```python
from build123d import *

# Parameters (mm, degrees)
F0_R          = 40
F1_DEPTH      = 20
F2_W          = 11
F2_H          = 10
F3_DEPTH      = 50
F3_DEPTH_BACK = 10
F4_R          = 6
F6_DEPTH      = 5
F7_R          = 6.4
F8_DEPTH      = 25
F9_R          = 1.5
F10_DEPTH     = 16
F11_R         = 3
F12_DEPTH     = 6


# Not quite as in the source:
# - a pattern or mirror of a feature is missing from the dataset's text; its kind, count and spacing are read off the source's solid


with BuildPart() as f1:
    # F0 (on Front) → F1 (new body)
    with BuildSketch(Plane.XZ):
        Circle(F0_R)
    extrude(amount=F1_DEPTH)

    # F2 (on Right) → F3 (cut, two sides)
    with BuildSketch(Plane.YZ) as f3_sk:
        with Locations((-5.5, 29)):
            Rectangle(F2_W, F2_H)
    f3 = extrude(amount=F3_DEPTH, mode=Mode.SUBTRACT) + extrude(f3_sk.sketch, amount=-F3_DEPTH_BACK, mode=Mode.SUBTRACT)

    # F3_copies: F3 across plane
    add(f3.mirror(Plane(origin=(0, 0, 0), x_dir=(-1, 0, 0), z_dir=(0, 0, -1))), mode=Mode.SUBTRACT)

    # F4
    f4_edges = [f1.edges().sort_by_distance(p)[0] for p in [
        (-40, -20, 0),
    ]]
    fillet(f4_edges, radius=F4_R)

    # F5 (on face) → F6 (cut)
    with BuildSketch(Plane.XZ.offset(20)):
        Polygon((-5.715767665, -9.9), (5.715767665, -9.9), (11.43153533, 0), (5.715767665, 9.9), (-5.715767665, 9.9), (-11.43153533, 0), align=None)
    extrude(amount=-F6_DEPTH, mode=Mode.SUBTRACT)

    # F7 (on face) → F8 (cut)
    with BuildSketch(Plane.XZ.offset(15)):
        Circle(F7_R)
    extrude(amount=-F8_DEPTH, mode=Mode.SUBTRACT)

    # F9 (on Front) → F10 (cut)
    with BuildSketch(Plane.XZ):
        with Locations((26, 12)):
            Circle(F9_R)
        with Locations((-26, 12)):
            Circle(F9_R)
        with Locations((-26, -12)):
            Circle(F9_R)
        with Locations((26, -12)):
            Circle(F9_R)
    extrude(amount=F10_DEPTH, mode=Mode.SUBTRACT)

    # F11 (on face) → F12 (cut)
    with BuildSketch(Plane(origin=(0, 0, 0), x_dir=(-1, 0, 0), z_dir=(0, 1, 0))):
        with Locations((-26, 12)):
            Circle(F11_R)
        with Locations((26, 12)):
            Circle(F11_R)
        with Locations((26, -12)):
            Circle(F11_R)
        with Locations((-26, -12)):
            Circle(F11_R)
    extrude(amount=-F12_DEPTH, mode=Mode.SUBTRACT)


solid = f1.part
```
The listing builds one solid part. Answer for the finished solid, in the listing's coordinates (mm). A direction names the side the tool comes from. Coordinates: 2 decimals unless noted, no trailing zeros. Loops run counter-clockwise (first coordinate to the right, second up) from the corner with the lowest first, then second, coordinate; pieces in that order, holes last. Notation, with made-up numbers: (3.25, -25.5) -> (21.25, -25.5) arc R34 cw to (21.25, 8.5) -> close; hole circle Ø6 at (87.25, 9). An arc over 180 degrees is marked (long way). Return JSON: item names as keys, results as strings. Group by question number.
(1) Which of the six approach directions +Z, -Z, +X, -X, +Y, -Y give full straight-line access (tool end or side, diameter ignored) to faces 1 (the cylindrical face through (-5.08, -7.6, -3.89)), 2 (the flat face through (11, -6, -24)), 3 (the flat face through (-1, 0, -8)), 4 (the flat face through (8.534, -17.535, -5.019)), 5 (the cylindrical face through (-27.5, -10.93, -11.93))?
(2) Given pin 1 Ø2.5 at (x, z) = (-26, 12) entering from +Y; pin 2 Ø3.5 at (x, z) = (26, 12) entering from +Y; pin 3 Ø3 at (x, z) = (14.5, -26.5) entering from +Y, each flat-ended and moving along its own axis, determine where each tip first touches the part or whether it passes through.
(3) Determine the mould class of faces 6 (the flat face through (24.7, -6, -13.3)), 7 (the flat face through (-10, -6, -29)), 8 (the flat face through (7, -20, 8)) for opening direction X: released by +X, released by -X, zero draft, split by the parting line, or undercut.
(4) A cutting plane is placed at A-A on x = 0. Write down the section's boundary in (y, z).
(5) Find the intervals of material crossed by probe 1 along Z at (x, y) = (26, -3.05); probe 2 along Z at (x, y) = (-4, -4); probe 3 along X at (y, z) = (-14, 12), in increasing order. Write a range as from..to.
(6) A cutting plane is placed at B-B on y = -9.5. Write down the section's boundary in (x, z).
The answers:
{
 "1": {"face 1": "+Y, -Y", "face 2": "+X, +Y", "face 3": "+Z, -Z, +X, -X, +Y", "face 4": "-Y", "face 5": "+Y"},
 "2": {"pin 1": "stops at y = -16", "pin 2": "stops at y = -6", "pin 3": "stops at y = -11"},
 "3": {"face 6": "undercut", "face 7": "released by +X", "face 8": "zero draft"},
 "4": {"outline": "(-20, -34) arc R6 ccw to (-14, -40) -> (0, -40) -> (0, -34) -> (-11, -34) -> (-11, -24) -> (0, -24) -> (0, -6.4) -> (-15, -6.4) -> (-15, -9.9) -> (-20, -9.9) -> close; (-20, 9.9) -> (-15, 9.9) -> (-15, 6.4) -> (0, 6.4) -> (0, 24) -> (-11, 24) -> (-11, 34) -> (0, 34) -> (0, 40) -> (-14, 40) arc R6 ccw to (-20, 34) -> close"},
 "5": {"probe 1": "z = -24..-15, -9..9, 15..24", "probe 2": "z = -39.8..-34, -24..-5, 5..24, 34..39.8", "probe 3": "x = -38.16..-27.5, -24.5..24.5, 27.5..38.16"},
 "6": {"outline": "(-10, -34) -> (-10, -24) -> (32, -24) arc R40 ccw to (32, 24) -> (-10, 24) -> (-10, 34) -> (21.07, 34) arc R40 ccw (long way) to (21.07, -34) -> close; hole circle Ø3 at (-26, -12); hole circle Ø3 at (-26, 12); hole circle Ø12.8 at (0, 0); hole circle Ø3 at (26, -12); hole circle Ø3 at (26, 12)"}
}
